```python
from build123d import *

# Parameters (mm, degrees)
F0_W     = 50
F0_H     = 80
F7_DEPTH = 25
F1_SIZE  = 5
F2_T     = -1
F3_R     = 6.6975560133
F3_R_2   = 3.0346294706
F4_DEPTH = 10.92156
F6_D     = 4.4


with BuildPart() as f7:
    # F0 (on Top) → F7 (new body)
    with BuildSketch(Plane.XY):
        with Locations((25, 40)):
            Rectangle(F0_W, F0_H)
    extrude(amount=F7_DEPTH)

    # F1
    f1_edges = [f7.edges().sort_by_distance(p)[0] for p in [
        (50, 0, 12.5),
        (50, 40, 25),
        (25, 0, 25),
    ]]
    chamfer(f1_edges, length=F1_SIZE)

    # F2
    f2_openings = [f7.faces().sort_by_distance(p)[0] for p in [
        (0, 40.24109, 12.431866),
        (24.76431, 80, 12.390572),
    ]]
    offset(amount=F2_T, openings=f2_openings)

    # F3 (on face) → F4 (join)
    with BuildSketch(Plane.XY.offset(25)):
        with BuildLine():
            Line((33.1360828131, 35.084836185), (26.6411228282, 59.4008081287))
            ThreePointArc((26.6411228282, 59.4008081287), (20.3049834818, 64.2666572246), (13.9688441353, 59.4008081287))
            Line((13.9688441353, 59.4008081287), (7.4738841504, 35.084836185))
            ThreePointArc((7.4738841504, 35.084836185), (20.3049834818, 18.3766251965), (33.1360828131, 35.084836185))
        make_face()
        with Locations((20.3049834818, 31.6575630777)):
            Circle(F3_R, mode=Mode.SUBTRACT)
        with Locations((20.3049834818, 57.7083826065)):
            Circle(F3_R_2, mode=Mode.SUBTRACT)
    extrude(amount=F4_DEPTH)

    # F6 (through all)
    with Locations(Plane.YZ.offset(50)):
        with Locations((10, 15), (30, 15), (30, 5), (10, 5)):
            Hole(F6_D / 2)


solid = f7.part
```
Work out the finished part from the listing and answer in its coordinate system (mm). A direction names the side the tool comes from. Give positions to 0.01 mm unless a question says otherwise; leave off trailing zeros. Loops run counter-clockwise (first coordinate to the right, second up) from the corner with the lowest first, then second, coordinate; pieces in that order, holes last. Notation, with made-up numbers: (17.5, -10.75) -> (55.5, -10.75) arc R29 cw to (55.5, 25.25) -> close; hole circle Ø8 at (72.5, 39). An arc over 180 degrees is marked (long way). Write item = value, one per line. Start each with the question number.
(1) Which of the six approach directions +Z, -Z, +X, -X, +Y, -Y give full straight-line access (tool end or side, diameter ignored) to faces 4 (the flat face through (49, 42, 10)), 5 (the flat face through (10.767, 47.413, 30.384)), 6 (the cylindrical face through (20.425, 64.266, 30.384)), 7 (the flat face through (20, 32, 25))?
(2) The mould has two halves that part along X. Classify faces 1 (the flat face through (26.7, 80, 24.5)), 2 (the flat face through (0, 39.8, 0.4)), 3 (the cylindrical face through (19.433, 38.298, 30.384)): +X half, -X half, draft (parallel to the pull), parting line (faces both ways), or undercut.
(3) Given pin 1 Ø5.5 at (y, z) = (30, 15) entering from -X; pin 2 Ø6 at (y, z) = (56.5, 30) entering from -X; pin 3 Ø20.5 at (x, z) = (23.5, 11.5) entering from +Y, each flat-ended and moving along its own axis, determine where each tip first touches the part or whether it passes through.
(4) Find section C-C on x = 42. Give the vertices of the cut face in (y, z), and give its area (3 significant figures).
(5) Find the intervals of material crossed by probe 1 along Z at (x, y) = (27, 19.5); probe 2 along Z at (x, y) = (31, 34); probe 3 along X at (y, z) = (11, 11), in increasing order. Write a range as from..to.
(6) Find section B-B on z = 15. Give the vertices of the cut face in (x, y), and give its area (3 significant figures).
(7) Find section D-D on z = 28. Give the vertices of the cut face in (x, y), and give its area (3 significant figures).
(8) Find section A-A on y = 10. Give the vertices of the cut face in (x, z).
From the geometry:
q1.face_4 = -X, +Y
q1.face_5 = +Z, -X, +Y
q1.face_6 = +Z, +Y
q1.face_7 = +Z
q2.face_1 = draft
q2.face_2 = -X half
q2.face_3 = undercut
q3.pin_1 = 49
q3.pin_2 = 12.39
q3.pin_3 = 3.16
q4.outline = (0, 0) -> (80, 0) -> (80, 1) -> (1, 1) -> (1, 19.59) -> (5.41, 24) -> (80, 24) -> (80, 25) -> (5, 25) -> (0, 20) -> close
q4.area = 180 mm^2
q5.probe_1 = 0..1, 24..25
q5.probe_2 = 0..1, 24..35.92
q5.probe_3 = 49..50
q6.outline = (0, 0) -> (45, 0) -> (50, 5) -> (50, 7.8) -> (49, 7.8) -> (49, 5.41) -> (44.59, 1) -> (0, 1) -> close; (49, 12.2) -> (50, 12.2) -> (50, 27.8) -> (49, 27.8) -> close; (49, 32.2) -> (50, 32.2) -> (50, 80) -> (49, 80) -> close
q6.area = 117 mm^2
q7.outline = (7.47, 35.08) arc R13.28 ccw (long way) to (33.14, 35.08) -> (26.64, 59.4) arc R6.56 ccw to (13.97, 59.4) -> close; hole circle Ø13.4 at (20.3, 31.66); hole circle Ø6.07 at (20.3, 57.71)
q7.area = 709 mm^2
q8.outline = (0, 0) -> (50, 0) -> (50, 2.8) -> (49, 2.8) -> (49, 1) -> (0, 1) -> close; (0, 24) -> (44.59, 24) -> (49, 19.59) -> (49, 17.2) -> (50, 17.2) -> (50, 20) -> (45, 25) -> (0, 25) -> close; (49, 7.2) -> (50, 7.2) -> (50, 12.8) -> (49, 12.8) -> close
